Geometry: final body of the model. Coordinates: model frame, mm. Give positions to 0.01 mm unless a question says otherwise; leave off trailing zeros. Write each loop counter-clockwise with the first axis right and the second up, starting at its lowest first coordinate (ties: lowest second). Pieces come first, ordered by that corner, then holes. Notation, with made-up numbers: M 33,83.5 L 86,83.5 A20 cw 86,103.5 Z; hole C 52,-2 d9. An arc over 180 degrees is marked long. One line per question, with ' | ' between items.
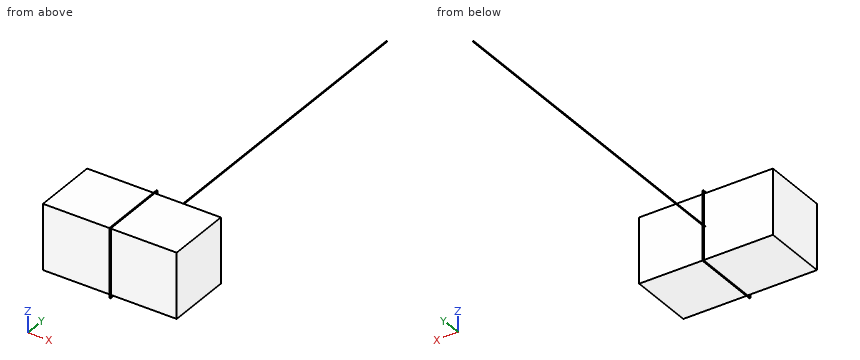
from build123d import *

# Parameters (mm, degrees)
SKETCH1_W                = 198.4375
SKETCH1_H                = 96.8375
EXTRUDE1_DEPTH           = 48.41875
ESBO_O2_R                = 0.714449934
ESBO_O3_R                = 0.635
RESSALTO_EXTRUS_O1_DEPTH = 508


with BuildPart() as part:
    # Sketch1 → Extrude1 (new body, symmetric)
    with BuildSketch(Plane.XY):
        with Locations((99.21875, -48.41875)):
            Rectangle(SKETCH1_W, SKETCH1_H)
    extrude(amount=EXTRUDE1_DEPTH, both=True)



with BuildPart() as body_2:
    # Varredura1: sweep along a path in Esbo_o1
    with BuildLine(Plane(origin=(101.6, 0, 0), x_dir=(0, 0, -1), z_dir=(1, 0, 0))) as varredura1_path:
        Line((-50.95875, 2.54), (50.95875, 2.54))
        Line((50.95875, 2.54), (50.95875, -99.3775))
        Line((50.95875, -99.3775), (-50.95875, -99.3775))
        Line((-50.95875, -99.3775), (-50.95875, 2.54))
    # Esbo_o2 → Varredura1 (sweep)
    with BuildSketch(Plane.XY):
        with Locations((101.6, 2.54)):
            Circle(ESBO_O2_R)
    sweep(path=varredura1_path.line, transition=Transition.RIGHT)


with BuildPart() as part_1:
    add(part.part)

    add(body_2.part)  # Ressalto-extrus_o1 merges body 2
    # Esbo_o3 → Ressalto-extrus_o1 (add)
    with BuildSketch(Plane(origin=(0, 0, 0), x_dir=(1, 0, 0), z_dir=(0, 1, 0))):
        with Locations((100.885550066, 0)):
            Circle(ESBO_O3_R)
    extrude(amount=RESSALTO_EXTRUS_O1_DEPTH)


solid = part_1.part
(1) Cut plane B-B, the plane y = -14.5. Return loops of the section in (x, z), then the cut area to 3 significant figures.
Working result:
outline: M 0,-48.42 L 198.44,-48.42 L 198.44,48.42 L 0,48.42 Z; C 101.6,-50.96 d1.43; C 101.6,50.96 d1.43 | area: 19,200 mm^2
(2) Cut plane A-A, the plane z = -26. Return loops of the section in (x, y).
Working result:
outline: M 0,-96.84 L 198.44,-96.84 L 198.44,0 L 0,0 Z; C 101.6,-99.38 d1.43; C 101.6,2.54 d1.43
(3) Cut plane D-D, the plane y = 376.5. Return loops of the section in (x, z) (3 decimals).
Working result:
outline: C 100.886,0 d1.27
(4) First-contact query: P1, Ø1, axis at x = 21, z = -1.5, coming from the -Y side; P2, Ø6, axis at x = 26, z = 13.5, coming from the +Y side. Flat tips, straight axial feed; report the tip coordinate or a pass-through.
Working result:
P1: stops at y = -96.84 | P2: stops at y = 0
(5) Material intervals for L1, parallel to Y at x = 54, z = 44.5; L2, parallel to Z at x = 95, y = -22, sorted ascending. Write a range as [from, to].
Working result:
L1: y = [-96.84, 0] | L2: z = [-48.42, 48.42]
(6) Cut plane C-C, the plane x = 135.5. Return loops of the section in (y, z).
Working result:
outline: M -96.84,-48.42 L 0,-48.42 L 0,48.42 L -96.84,48.42 Z
